from build123d import *

# Parameters (mm, degrees)
EXTRUDE_1_DEPTH      = 125
EXTRUDE_1_DEPTH_BACK = 125
SHELL_1_T            = -3
CHAMFER_1_SIZE       = 5.358983849
CHAMFER_1_SIZE_2     = 20


with BuildPart() as part:
    # Эскиз1 → Бобышка-Вытянуть1 (new, two sides: drawn at the far end of the back side and taken through both)
    with BuildSketch(Plane.XY.offset(-EXTRUDE_1_DEPTH_BACK)):
        with BuildLine():
            Line((-14, 10), (14, 10))
            ThreePointArc((14, 10), (18.242640687, 8.242640687), (20, 4))
            Line((20, 4), (20, -4))
            ThreePointArc((20, -4), (18.242640687, -8.242640687), (14, -10))
            Line((14, -10), (-14, -10))
            ThreePointArc((-14, -10), (-18.242640687, -8.242640687), (-20, -4))
            Line((-20, -4), (-20, 4))
            ThreePointArc((-20, 4), (-18.242640687, 8.242640687), (-14, 10))
        make_face()
    extrude(amount=EXTRUDE_1_DEPTH + EXTRUDE_1_DEPTH_BACK)

    # Оболочка1
    shell_1_openings = [part.faces().sort_by_distance(p)[0] for p in [
        (0, 0, -125),
        (0, 0, 125),
    ]]
    offset(amount=SHELL_1_T, openings=shell_1_openings, kind=Kind.INTERSECTION)

    # Фаска1
    # the kernel refuses this chamfer: 20, 5.358983849 mm, written as the material it takes off along each edge
    with BuildSketch(Plane(origin=(-65.934431404, 10, -125), x_dir=(0, 0.13751244702128945, 0.9905000388259543), z_dir=(1, 0, 0))) as chamfer_1_piece_1:
        Polygon((CHAMFER_1_SIZE * 0.990500038756, CHAMFER_1_SIZE * 0.137512447012), (-CHAMFER_1_SIZE_2 * 0.137512447021, CHAMFER_1_SIZE_2 * 0.990500038826), (0, 0), align=None)
    extrude(amount=131.868862808, mode=Mode.SUBTRACT)
    with BuildSketch(Plane(origin=(-65.934431404, 10, 125), x_dir=(0, 0.13751244702128945, -0.9905000388259543), z_dir=(1, 0, 0))) as chamfer_1_piece_2:
        Polygon((CHAMFER_1_SIZE * 0.990500038756, -CHAMFER_1_SIZE * 0.137512447012), (-CHAMFER_1_SIZE_2 * 0.137512447021, -CHAMFER_1_SIZE_2 * 0.990500038826), (0, 0), align=None)
    extrude(amount=131.868862808, mode=Mode.SUBTRACT)


solid = part.part
Design review of the part built by this model. Coordinates are the model's own, in mm. A direction names the side the tool comes from. Round coordinates to 2 decimals unless told otherwise and drop trailing zeros. Write each loop counter-clockwise with the first axis right and the second up, starting at its lowest first coordinate (ties: lowest second). Pieces come first, ordered by that corner, then holes.
Item 1: Wall thickness on L1, parallel to Y at x = -7, z = 113; L2, parallel to X at y = -0.25, z = -112; L3, parallel to Y at x = -15, z = 60: over which ranges is each line inside the solid? List them lowest first.
Item 2: Consider section A-A on x = -2. Give the boundary of the cut face in (y, z), and give its area (3 significant figures).
Item 3: Consider section B-B on z = 96. Give the boundary of the cut face in (x, y).
Item 4: For faces 4 (the flat face through (0, -7, -2)), 5 (the flat face through (0, -10, -2)), list the 3-axis set-ups (+Z, -Z, +X, -X, +Y, -Y) from which the entire face can be reached by the end or side of a thin tool; tool diameter is ignored.
Item 5: For pin 1 Ø1.5 at (x, y) = (-13.5, -8) entering from -Z, flat-tipped, find the tip position at first contact; note if it passes through.
Item 6: Draft analysis for pull direction Y (two halves, no side actions). For faces 1 (the cylindrical face through (18.289, -8.196, -1.75)), 2 (the flat face through (-0.093, 7.454, -120.323)), 3 (the flat face through (-17, 0, -2)), state which applies: released by +Y, released by -Y, zero draft, split by the parting line, or undercut.
Check values:
1. L1: y = -10 to -7, 7 to 10
1. L2: x = -20 to -17, 17 to 20
1. L3: y = -9.92 to -6.83, 6.83 to 9.92
2. outline: (-10, -125) - (-7, -124.2) - (-7, 124.2) - (-10, 125) - close; (7, -120.44) - (10, -119.64) - (10, 119.64) - (7, 120.44) - close
2. area: 1,470 mm2
3. outline: (-20, -4) arc R6 ccw to (-14, -10) - (14, -10) arc R6 ccw to (20, -4) - (20, 4) arc R6 ccw to (14, 10) - (-14, 10) arc R6 ccw to (-20, 4) - close; hole (-17, -4) arc R3 ccw to (-14, -7) - (14, -7) arc R3 ccw to (17, -4) - (17, 4) arc R3 ccw to (14, 7) - (-14, 7) arc R3 ccw to (-17, 4) - close
4. face 4: +Z, -Z
4. face 5: +Z, -Z, +X, -X, -Y
5. pin 1: stops at z = -124.67
6. face 1: released by -Y
6. face 2: released by +Y
6. face 3: undercut
